Geometry: see drawing. Coordinates: mm, zero at the bounding-box minimum. A direction names the side the tool comes from. Give positions to 0.01 mm unless a question says otherwise; leave off trailing zeros. Write each loop counter-clockwise with the first axis right and the second up, starting at its lowest first coordinate (ties: lowest second). Pieces come first, ordered by that corner, then holes. Notation, with made-up numbers: (6.5, 1) -> (46.5, 1) arc R31 cw to (46.5, 38) -> close; hole circle Ø8 at (-6.75, -3.75). An arc over 180 degrees is marked (long way). Answer as a JSON object with one key per item and string values. Group by question number.
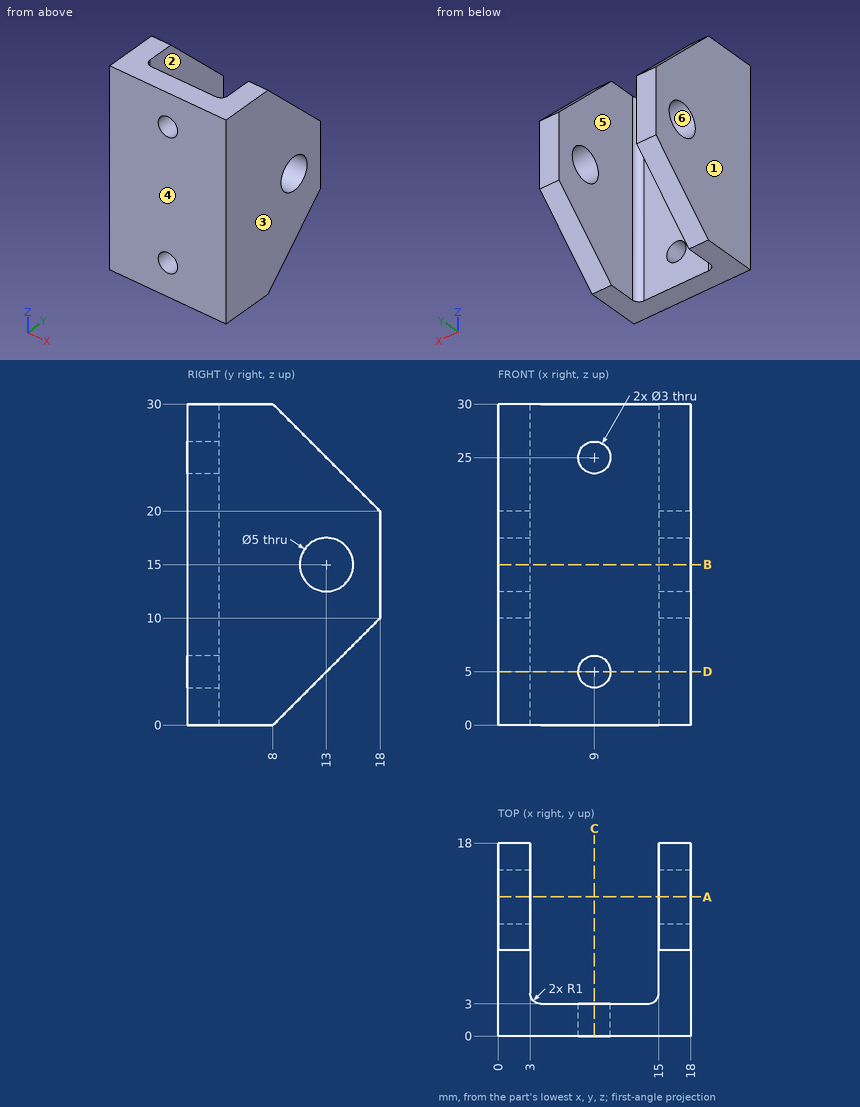
1. Section A-A (y = 13). Return the cut outline in (x, z), plus the area to 3 significant figures.
2. Reachability of the marked faces 5 and 6 from +Z, -Z, +X, -X, +Y, -Y: full face, straight path, thin tool, end or side. Return the list, or none.
3. Mould query, pull axis X, two halves, no side actions, for the marked faces 1, 2, 3 and 4. Classes: pulls with the +X half, pulls with the -X half, needs draft (parallel to the pull), parting line crosses it, or undercut.
4. Section C-C (x = 9). Return the cut outline in (y, z), plus the area to 3 significant figures.
5. Contact query for flat-ended pins moving along their axis: pin 1 Ø1.5 at (x, y) = (4.5, 11) entering from +Z; pin 2 Ø3 at (x, z) = (15, 5) entering from +Y; pin 3 Ø3.5 at (x, z) = (9, 5) entering from +Y. Output: stop coordinate, or through.
6. Line query: line 1 (X direction, y = 12.5, z = 8.25); line 2 (X direction, y = 2.45, z = 25); line 3 (Y direction, x = 9.5, z = 14). Output: solid intervals per line, ascending.
7. Section B-B (z = 15). Return the cut outline in (x, y).
8. Section D-D (z = 5). Return the cut outline in (x, y), plus the area to 3 significant figures.
Working result:
{
 "1": {"outline": "(0, 5) -> (3, 5) -> (3, 12.5) -> (0, 12.5) -> close; (0, 17.5) -> (3, 17.5) -> (3, 25) -> (0, 25) -> close; (15, 5) -> (18, 5) -> (18, 12.5) -> (15, 12.5) -> close; (15, 17.5) -> (18, 17.5) -> (18, 25) -> (15, 25) -> close", "area": "90.0 mm^2"},
 "2": {"face 5": "+Z, -Z, +Y", "face 6": "+X, -X"},
 "3": {"face 1": "pulls with the -X half", "face 2": "undercut", "face 3": "pulls with the +X half", "face 4": "needs draft"},
 "4": {"outline": "(0, 0) -> (3, 0) -> (3, 3.5) -> (0, 3.5) -> close; (0, 6.5) -> (3, 6.5) -> (3, 23.5) -> (0, 23.5) -> close; (0, 26.5) -> (3, 26.5) -> (3, 30) -> (0, 30) -> close", "area": "72.0 mm^2"},
 "5": {"pin 1": "passes through", "pin 2": "stops at y = 14.5", "pin 3": "stops at y = 3"},
 "6": {"line 1": "x = 0 to 3, 15 to 18", "line 2": "x = 0 to 7.5, 10.5 to 18", "line 3": "y = 0 to 3"},
 "7": {"outline": "(0, 0) -> (18, 0) -> (18, 10.5) -> (15, 10.5) -> (15, 4) arc R1 cw to (14, 3) -> (4, 3) arc R1 cw to (3, 4) -> (3, 10.5) -> (0, 10.5) -> close; (0, 15.5) -> (3, 15.5) -> (3, 18) -> (0, 18) -> close; (15, 15.5) -> (18, 15.5) -> (18, 18) -> (15, 18) -> close"},
 "8": {"outline": "(0, 0) -> (7.5, 0) -> (7.5, 3) -> (4, 3) arc R1 cw to (3, 4) -> (3, 13) -> (0, 13) -> close; (10.5, 0) -> (18, 0) -> (18, 13) -> (15, 13) -> (15, 4) arc R1 cw to (14, 3) -> (10.5, 3) -> close", "area": "105 mm^2"}
}
